Build history of the part. All positions in model axes, mm. A direction names the side the tool comes from. Coordinates: 2 decimals unless noted, no trailing zeros. Write each loop counter-clockwise with the first axis right and the second up, starting at its lowest first coordinate (ties: lowest second). Pieces come first, ordered by that corner, then holes.
from build123d import *

# Parameters (mm, degrees)
SKETCH1_R           = 7
BOSS_EXTRUDE1_DEPTH = 9
CUT_EXTRUDE1_START  = -2
SKETCH2_R           = 8
CUT_EXTRUDE1_DEPTH  = 2


with BuildPart() as part:
    # Sketch1 → Boss-Extrude1 (new body)
    with BuildSketch(Plane.XY):
        with BuildLine():
            Line((-191.078194945, -17.5), (-144.521304841, -17.5))
            ThreePointArc((-144.521304841, -17.5), (-142.399984498, -16.621320344), (-141.521304841, -14.5))
            Line((-141.521304841, -14.5), (-141.521304841, 14.5))
            ThreePointArc((-141.521304841, 14.5), (-142.399984498, 16.621320344), (-144.521304841, 17.5))
            Line((-144.521304841, 17.5), (-191.078194945, 17.5))
            ThreePointArc((-191.078194945, 17.5), (-193.199515288, 16.621320344), (-194.078194945, 14.5))
            Line((-194.078194945, 14.5), (-194.078194945, -14.5))
            ThreePointArc((-194.078194945, -14.5), (-193.199515288, -16.621320344), (-191.078194945, -17.5))
        make_face()
        with Locations((-185.692771804, 0)):
            Circle(SKETCH1_R, mode=Mode.SUBTRACT)
        with BuildLine():
            Line((-178.368092358, 10.25), (-186.368092358, 10.25))
            ThreePointArc((-186.368092358, 10.25), (-188.368092358, 12.25), (-186.368092358, 14.25))
            Line((-186.368092358, 14.25), (-178.368092358, 14.25))
            ThreePointArc((-178.368092358, 14.25), (-176.368092358, 12.25), (-178.368092358, 10.25))
        make_face(mode=Mode.SUBTRACT)
        with BuildLine():
            Line((-151.521304841, -14.25), (-159.521304841, -14.25))
            ThreePointArc((-159.521304841, -14.25), (-161.521304841, -12.25), (-159.521304841, -10.25))
            Line((-159.521304841, -10.25), (-151.521304841, -10.25))
            ThreePointArc((-151.521304841, -10.25), (-149.521304841, -12.25), (-151.521304841, -14.25))
        make_face(mode=Mode.SUBTRACT)
        with BuildLine():
            Line((-151.521304841, 10.25), (-159.521304841, 10.25))
            ThreePointArc((-159.521304841, 10.25), (-161.521304841, 12.25), (-159.521304841, 14.25))
            Line((-159.521304841, 14.25), (-151.521304841, 14.25))
            ThreePointArc((-151.521304841, 14.25), (-149.521304841, 12.25), (-151.521304841, 10.25))
        make_face(mode=Mode.SUBTRACT)
        with BuildLine():
            Line((-178.368092358, -14.25), (-186.368092358, -14.25))
            ThreePointArc((-186.368092358, -14.25), (-188.368092358, -12.25), (-186.368092358, -10.25))
            Line((-186.368092358, -10.25), (-178.368092358, -10.25))
            ThreePointArc((-178.368092358, -10.25), (-176.368092358, -12.25), (-178.368092358, -14.25))
        make_face(mode=Mode.SUBTRACT)
    extrude(amount=BOSS_EXTRUDE1_DEPTH)

    # Sketch2 → Cut-Extrude1 (cut)
    with BuildSketch(Plane.XY.offset(9).offset(CUT_EXTRUDE1_START)):
        with BuildLine():
            Line((-194.078194945, 14.5), (-194.078194945, -14.5))
            ThreePointArc((-194.078194945, -14.5), (-193.199515288, -16.621320344), (-191.078194945, -17.5))
            Line((-191.078194945, -17.5), (-144.521304841, -17.5))
            ThreePointArc((-144.521304841, -17.5), (-142.399984498, -16.621320344), (-141.521304841, -14.5))
            Line((-141.521304841, -14.5), (-141.521304841, 14.5))
            ThreePointArc((-141.521304841, 14.5), (-142.399984498, 16.621320344), (-144.521304841, 17.5))
            Line((-144.521304841, 17.5), (-191.078194945, 17.5))
            ThreePointArc((-191.078194945, 17.5), (-193.199515288, 16.621320344), (-194.078194945, 14.5))
        make_face()
        with Locations((-185.692771804, 0)):
            Circle(SKETCH2_R, mode=Mode.SUBTRACT)
        with BuildLine():
            ThreePointArc((-186.368092358, -14.25), (-188.368092358, -12.25), (-186.368092358, -10.25))
            Line((-186.368092358, -10.25), (-178.368092358, -10.25))
            ThreePointArc((-178.368092358, -10.25), (-176.368092358, -12.25), (-178.368092358, -14.25))
            Line((-178.368092358, -14.25), (-186.368092358, -14.25))
        make_face(mode=Mode.SUBTRACT)
        with BuildLine():
            Line((-151.521304841, -14.25), (-159.521304841, -14.25))
            ThreePointArc((-159.521304841, -14.25), (-161.521304841, -12.25), (-159.521304841, -10.25))
            Line((-159.521304841, -10.25), (-151.521304841, -10.25))
            ThreePointArc((-151.521304841, -10.25), (-149.521304841, -12.25), (-151.521304841, -14.25))
        make_face(mode=Mode.SUBTRACT)
        with BuildLine():
            ThreePointArc((-159.521304841, 10.25), (-161.521304841, 12.25), (-159.521304841, 14.25))
            Line((-159.521304841, 14.25), (-151.521304841, 14.25))
            ThreePointArc((-151.521304841, 14.25), (-149.521304841, 12.25), (-151.521304841, 10.25))
            Line((-151.521304841, 10.25), (-159.521304841, 10.25))
        make_face(mode=Mode.SUBTRACT)
        with BuildLine():
            Line((-186.368092358, 14.25), (-178.368092358, 14.25))
            ThreePointArc((-178.368092358, 14.25), (-176.368092358, 12.25), (-178.368092358, 10.25))
            Line((-178.368092358, 10.25), (-186.368092358, 10.25))
            ThreePointArc((-186.368092358, 10.25), (-188.368092358, 12.25), (-186.368092358, 14.25))
        make_face(mode=Mode.SUBTRACT)
    extrude(amount=CUT_EXTRUDE1_DEPTH, mode=Mode.SUBTRACT)


solid = part.part
(1) Slice it at C-C, the plane z = 1.5. List the corners of the cut face in (x, y).
(2) Slice it at A-A, the plane y = 0. List the corners of the cut face in (x, z), and give its area (3 significant figures).
(3) 3-axis set-ups, long thin cutter, end or side, ignore diameter. For faces 1 (the flat face through (-182, 10.25, 3)), 2 (the flat face through (-194.078, 0, 3)): which of +Z, -Z, +X, -X, +Y, -Y reach the whole face in a straight line?
(4) Slice it at B-B, the plane y = 12.25. List the corners of the cut face in (x, z), and give its area (3 significant figures).
(5) Flat gauge pins, fed straight in: P1, Ø12, axis at x = -158.5, y = -5.5, coming from the -Z side; P2, Ø3, axis at x = -185, y = 13.5, coming from the +Z side. Where does each tip first touch, or does it go through?
(6) Slice it at D-D, the plane z = 8. List the corners of the cut face in (x, y).
(7) Probe L1, parallel to Y at x = -158, z = 1.5; L2, parallel to X at y = 13, z = 1; L3, parallel to Y at x = -180, z = 2.5. List the from-to ranges inside material, lowest first.
(8) Two-plate mould, pull along X, no slides. Class faces 3 (the flat face through (-180, -5, 9)), 4 (the flat face through (-141.521, 0, 3)), 5 (the cylindrical face through (-161.52, 12.21, 3.45)): pulls with the +X half, pulls with the -X half, needs draft (parallel to the pull), parting line crosses it, or undercut.
Results:
1. outline: (-194.08, -14.5) arc R3 ccw to (-191.08, -17.5) - (-144.52, -17.5) arc R3 ccw to (-141.52, -14.5) - (-141.52, 14.5) arc R3 ccw to (-144.52, 17.5) - (-191.08, 17.5) arc R3 ccw to (-194.08, 14.5) - close; hole circle Ø14 at (-185.69, 0); hole (-186.37, -14.25) - (-178.37, -14.25) arc R2 ccw to (-178.37, -10.25) - (-186.37, -10.25) arc R2 ccw to start; hole (-186.37, 10.25) - (-178.37, 10.25) arc R2 ccw to (-178.37, 14.25) - (-186.37, 14.25) arc R2 ccw to start; hole (-159.52, -14.25) - (-151.52, -14.25) arc R2 ccw to (-151.52, -10.25) - (-159.52, -10.25) arc R2 ccw to start; hole (-159.52, 10.25) - (-151.52, 10.25) arc R2 ccw to (-151.52, 14.25) - (-159.52, 14.25) arc R2 ccw to start
2. outline: (-194.08, 0) - (-192.69, 0) - (-192.69, 9) - (-193.69, 9) - (-193.69, 7) - (-194.08, 7) - close; (-178.69, 0) - (-141.52, 0) - (-141.52, 7) - (-177.69, 7) - (-177.69, 9) - (-178.69, 9) - close
2. area: 274 mm2
3. face 1: +Z, -Z
3. face 2: +Z, -Z, -X, +Y, -Y
4. outline: (-194.08, 0) - (-188.37, 0) - (-188.37, 7) - (-194.08, 7) - close; (-176.37, 0) - (-161.52, 0) - (-161.52, 7) - (-176.37, 7) - close; (-149.52, 0) - (-141.52, 0) - (-141.52, 7) - (-149.52, 7) - close
4. area: 200 mm2
5. P1: stops at z = 0
5. P2: stops at z = 7
6. outline: circle Ø16 at (-185.69, 0); hole circle Ø14 at (-185.69, 0)
7. L1: y = -17.5 to -14.25, -10.25 to 10.25, 14.25 to 17.5
7. L2: x = -194.08 to -188.22, -176.51 to -161.38, -149.67 to -141.52
7. L3: y = -17.5 to -14.25, -10.25 to -4.07, 4.07 to 10.25, 14.25 to 17.5
8. face 3: needs draft
8. face 4: pulls with the +X half
8. face 5: undercut
